```python
from build123d import *

# Parameters (mm, degrees)
F1_DEPTH = 37
F2_R     = 1.5
F3_DEPTH = 12.001
F4_R     = 1.75
F5_DEPTH = 25.001
F6_R     = 8
F7_SIZE  = 2


with BuildPart() as f1:
    # F0 (on Right) → F1 (new body)
    with BuildSketch(Plane.YZ):
        Polygon((-12, 0), (0, 0), (0, 25), (-1.5, 25), (-1.5, 1.5), (-12, 1.5), align=None)
    extrude(amount=-F1_DEPTH)

    # F2 (on Front) → F3 (cut, through all)
    with BuildSketch(Plane.XZ):
        with Locations((-33.2, 18.727851)):
            Circle(F2_R)
        with Locations((-19.62, 8.062404)):
            Circle(F2_R)
    extrude(amount=F3_DEPTH, mode=Mode.SUBTRACT)

    # F4 (on Top) → F5 (cut, through all)
    with BuildSketch(Plane.XY):
        with Locations((-5, -7)):
            Circle(F4_R)
        with Locations((-17, -7)):
            Circle(F4_R)
    extrude(amount=F5_DEPTH, mode=Mode.SUBTRACT)

    # F6
    f6_edges = [f1.edges().sort_by_distance(p)[0] for p in [
        (-37, -12, 0.75),
    ]]
    fillet(f6_edges, radius=F6_R)

    # F7
    f7_edges = [f1.edges().sort_by_distance(p)[0] for p in [
        (-37, -0.75, 25),
        (0, -0.75, 25),
    ]]
    chamfer(f7_edges, length=F7_SIZE)


solid = f1.part
```
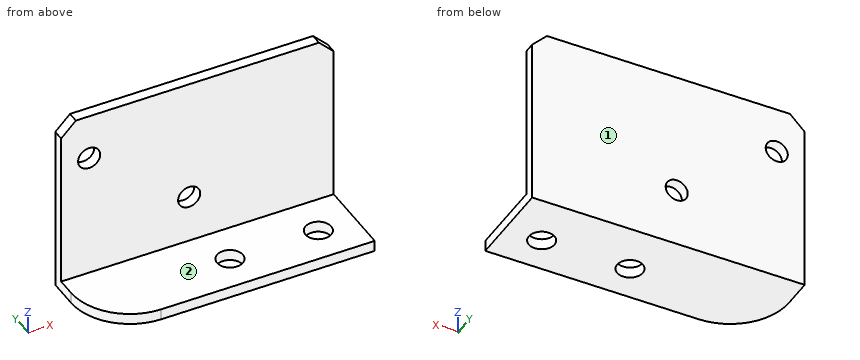
Check sheet for the modelled part. Datum: model origin and axes. Units: mm. Face numbers are marked on the shaded views. A direction names the side the tool comes from. Round coordinates to 2 decimals unless told otherwise and drop trailing zeros. Loops run counter-clockwise (first coordinate to the right, second up) from the corner with the lowest first, then second, coordinate; pieces in that order, holes last. Notation, with made-up numbers: (-20.5, -1) - (10.5, -1) arc R30 cw to (10.5, 24) - close; hole circle Ø2 at (59, -11). An arc over 180 degrees is marked (long way). Answer as a JSON object with one key per item and string values. Group by question number.
Q1. Sectioned sample at A-A, the plane x = -5. Enter the section's corners in (y, z), plus the area to 3 significant figures.
Q2. Set-up check for the marked faces 1 and 2: record each of +Z, -Z, +X, -X, +Y, -Y from which the full face is reachable in a straight line by a thin tool's end or side.
Q3. Sectioned sample at B-B, the plane y = -5.75. Enter the section's corners in (x, z), plus the area to 3 significant figures.
Q4. Gauge pin test, flat ends, axial feed: P1, Ø2.5, axis at x = -33.2, z = 18.73, coming from the -Y side; P2, Ø1, axis at x = -21.5, y = -5.5, coming from the +Z side; P3, Ø12, axis at x = -23.5, z = 19, coming from the -Y side. Record the tip position at first contact, or that the pin passes through.
Q5. Sectioned sample at C-C, the plane z = 18.25. Enter the section's corners in (x, y), plus the area to 3 significant figures.
Q6. Sectioned sample at D-D, the plane x = -19.62. Enter the section's corners in (y, z).
Q7. Scan lines: line 1 along Y through (x, z) = (-17, 0.8); line 2 along Z through (x, y) = (-33.2, -0.85); line 3 along X through (y, z) = (-7, 0.65). Record each from-to range of solid material in increasing order. Write a range as [from, to].
Solution:
{
 "1": {"outline": "(-12, 0) - (-8.75, 0) - (-8.75, 1.5) - (-12, 1.5) - close; (-5.25, 0) - (0, 0) - (0, 25) - (-1.5, 25) - (-1.5, 1.5) - (-5.25, 1.5) - close", "area": "48.0 mm²"},
 "2": {"face 1": "+Z, -Z, +X, -X, +Y", "face 2": "+Z, +X, -X, -Y"},
 "3": {"outline": "(-36.81, 0) - (-18.22, 0) - (-18.22, 1.5) - (-36.81, 1.5) - close; (-15.78, 0) - (-6.22, 0) - (-6.22, 1.5) - (-15.78, 1.5) - close; (-3.78, 0) - (0, 0) - (0, 1.5) - (-3.78, 1.5) - close", "area": "47.9 mm²"},
 "4": {"P1": "passes through", "P2": "stops at z = 1.5", "P3": "stops at y = -1.5"},
 "5": {"outline": "(-37, -1.5) - (-34.62, -1.5) - (-34.62, 0) - (-37, 0) - close; (-31.78, -1.5) - (0, -1.5) - (0, 0) - (-31.78, 0) - close", "area": "51.2 mm²"},
 "6": {"outline": "(-12, 0) - (0, 0) - (0, 6.56) - (-1.5, 6.56) - (-1.5, 1.5) - (-12, 1.5) - close; (-1.5, 9.56) - (0, 9.56) - (0, 25) - (-1.5, 25) - close"},
 "7": {"line 1": "y = [-12, -8.75], [-5.25, 0]", "line 2": "z = [0, 17.23], [20.23, 25]", "line 3": "x = [-36.42, -18.75], [-15.25, -6.75], [-3.25, 0]"}
}
